Could you check a few things on this model? Use its own coordinates, in mm. A direction names the side the tool comes from. Give positions to 0.01 mm unless a question says otherwise; leave off trailing zeros. Write each loop counter-clockwise with the first axis right and the second up, starting at its lowest first coordinate (ties: lowest second). Pieces come first, ordered by that corner, then holes. Notation, with made-up numbers: M 88.25,73 L 96.25,73 A17 cw 96.25,88 Z; hole C 65,56 d7. An arc over 180 degrees is marked long. Answer as CSV lines item,"result". Start each with the question number.
from build123d import *

# Parameters (mm, degrees)
SKETCH1_W           = 64
SKETCH1_H           = 106.838
SKETCH1_W_2         = 60
SKETCH1_H_2         = 102.838
BOSS_EXTRUDE1_DEPTH = 2
SKETCH1_3_W         = 64
SKETCH1_3_H         = 106.838
SKETCH1_3_W_2       = 60
SKETCH1_3_H_2       = 102.838
BOSS_EXTRUDE2_DEPTH = 40


with BuildPart() as part:
    # Sketch1 → Boss-Extrude1 (new body)
    # profile 1 of 2: a face of its own
    with BuildSketch(Plane.XY):
        with Locations((32, 47)):
            Rectangle(SKETCH1_W, SKETCH1_H)
        with Locations((32, 47)):
            Rectangle(SKETCH1_W_2, SKETCH1_H_2, mode=Mode.SUBTRACT)
    # profile 2 of 2: a face of its own
    with BuildSketch(Plane.XY):
        with Locations((32, 47)):
            Rectangle(SKETCH1_W_2, SKETCH1_H_2)
    extrude(amount=BOSS_EXTRUDE1_DEPTH)

    # Sketch1_3 → Boss-Extrude2 (add)
    with BuildSketch(Plane.XY):
        with Locations((32, 47)):
            Rectangle(SKETCH1_3_W, SKETCH1_3_H)
        with Locations((32, 47)):
            Rectangle(SKETCH1_3_W_2, SKETCH1_3_H_2, mode=Mode.SUBTRACT)
    extrude(amount=BOSS_EXTRUDE2_DEPTH)


solid = part.part
1. Imagine slicing it at B-B, the plane y = 41.5. Please give me the cut outline in (x, z).
2. On a 3-axis mill with a long thin cutter (end or side, diameter ignored), from which of +Z, -Z, +X, -X, +Y, -Y can I reach the whole of each face in a straight line? I mean faces 1 (the flat face through (32, -4.419, 21)), 2 (the flat face through (64, 46, 20)). Say none if no direction works.
3. Imagine slicing it at A-A, the plane z = 17.5. Please give me the cut outline in (x, y), plus the area to 3 significant figures.
4. Will these pins go through, and if not, where does the flat tip stop? P1, Ø8, axis at x = 28.5, y = 66, coming from the -Z side; P2, Ø18, axis at x = 43, y = 58, coming from the +Z side.
5. Thinking about a two-plate mould opening in Y: for faces 3 (the flat face through (63, 63, 40)), 4 (the flat face through (32, -6.419, 20)), 5 (the flat face through (32, 48, 2)), which applies, pulls with the +Y half, pulls with the -Y half, needs draft (parallel to the pull), parting line crosses it, or undercut?
6. Please list where these lines run through material, in increasing order: line 1 (Y direction, x = 47.5, z = 12); line 2 (X direction, y = 58, z = 6.5); line 3 (Z direction, x = 8.5, y = 26).
7. Imagine slicing it at C-C, the plane x = 55.5. Please give me the cut outline in (y, z).
Solutions:
1,outline,"M 0,0 L 64,0 L 64,40 L 62,40 L 62,2 L 2,2 L 2,40 L 0,40 Z"
2,face 1,"+Z"
2,face 2,"+Z, -Z, +X, +Y, -Y"
3,outline,"M 0,-6.42 L 64,-6.42 L 64,100.42 L 0,100.42 Z; hole M 2,-4.42 L 62,-4.42 L 62,98.42 L 2,98.42 Z"
3,area,"667 mm²"
4,P1,"z = 0"
4,P2,"z = 2"
5,face 3,"needs draft"
5,face 4,"pulls with the -Y half"
5,face 5,"undercut"
6,line 1,"-6.42 to -4.42, 98.42 to 100.42"
6,line 2,"0 to 2, 62 to 64"
6,line 3,"0 to 2"
7,outline,"M -6.42,0 L 100.42,0 L 100.42,40 L 98.42,40 L 98.42,2 L -4.42,2 L -4.42,40 L -6.42,40 Z"
